```python
from build123d import *

# Parameters (mm, degrees)
SKETCH008_R          = 7.5
SKETCH008_R_2        = 6.6
PAD002_DEPTH         = 24
SKETCH009_R          = 9
SKETCH009_R_2        = 6.6
PAD003_DEPTH         = 2
POCKET006_DEPTH      = 81.774622
POCKET006_DEPTH_BACK = 81.774622
POLARPATTERN_COUNT   = 3


with BuildPart() as part:
    # Sketch008 (on DatumPlane) → Pad002 (new body)
    with BuildSketch(Plane.XZ.offset(50)):
        Circle(SKETCH008_R)
        Circle(SKETCH008_R_2, mode=Mode.SUBTRACT)
    extrude(amount=PAD002_DEPTH)

    # Sketch009 (on Face3 of Pad002) → Pad003 (join)
    with BuildSketch(Plane(origin=(0, -50, 0), x_dir=(1, 0, 0), z_dir=(0, 1, 0))):
        Circle(SKETCH009_R)
        Circle(SKETCH009_R_2, mode=Mode.SUBTRACT)
    extrude(amount=PAD003_DEPTH)

    # Sketch010 → Revolution (revolve)
    with BuildSketch(Plane.XY):
        Polygon((-7.5, -74), (-7.5, -71.3), (-8.7, -71.3), (-8.7, -72.3), (-7.7, -74), align=None)
    revolve(axis=Axis((0, 0, 0), (0, 1, 0)))

    # Sketch011 → Pocket006 (cut, two sides)
    with BuildSketch(Plane.XY) as pocket006_sk:
        with BuildLine():
            Line((-0.8, -74), (-0.8, -60))
            ThreePointArc((0.8, -60), (0, -59.2), (-0.8, -60))
            Line((0.8, -60), (0.8, -74))
            Line((-0.8, -74), (0.8, -74))
        make_face()
    pocket006 = extrude(amount=-POCKET006_DEPTH, mode=Mode.SUBTRACT) + extrude(pocket006_sk.sketch, amount=POCKET006_DEPTH_BACK, mode=Mode.SUBTRACT)

    # PolarPattern: Pocket006 ×3 about axis
    polarpattern_axis = Axis((0, 0, 0), (0, 1, 0))
    for i in range(1, POLARPATTERN_COUNT):
        add(pocket006.rotate(polarpattern_axis, i * 360 / POLARPATTERN_COUNT), mode=Mode.SUBTRACT)


solid = part.part
```
Geometry check sheet. Reference: the model listing, model coordinates, mm. A direction names the side the tool comes from. Round coordinates to 2 decimals unless told otherwise and drop trailing zeros. Order: outer loops, then holes, each group sorted by start corner. A loop starts at its lowest first (then second) coordinate and runs counter-clockwise, first axis right, second up. Notation, with made-up numbers: M 57.25,60 L 97.25,60 A26 ccw 97.25,86 Z; hole C 70,60 d7. An arc over 180 degrees is marked long. Write item = value, one per line.
Q1. Section check C-C (y = -64.25). Enter the section's corners in (x, z).
Answer block:
outline = M -6.86,-3.04 L -6.07,-2.58 A6.6 cw -6.07,2.58 L -6.86,3.04 A7.5 ccw Z; M -6.06,-4.42 A7.5 ccw -0.8,-7.46 L -0.8,-6.55 A6.6 cw -5.27,-3.97 Z; M -6.06,4.42 L -5.27,3.97 A6.6 cw -0.8,6.55 L -0.8,7.46 A7.5 ccw Z; M 0.8,-7.46 A7.5 ccw 6.06,-4.42 L 5.27,-3.97 A6.6 cw 0.8,-6.55 Z; M 0.8,6.55 A6.6 cw 5.27,3.97 L 6.06,4.42 A7.5 ccw 0.8,7.46 Z; M 6.07,-2.58 L 6.86,-3.04 A7.5 ccw 6.86,3.04 L 6.07,2.58 A6.6 cw Z
Q2. Set-up check for faces 5 (the flat face through (4, -71.3, -7)), 6 (the flat face through (-6.59, -68.46, -2.88)), 7 (the flat face through (0.8, -68, -7)): record each of +Z, -Z, +X, -X, +Y, -Y from which the full face is reachable in a straight line by a thin tool's end or side.
Answer block:
face_5 = -Z, +X
face_6 = -Y
face_7 = +Z, -Z, -Y
Q3. Section check D-D (y = -57). Enter the section's corners in (x, z), plus the area to 3 significant figures.
Answer block:
outline = C 0,0 d15; hole C 0,0 d13.2
area = 39.9 mm^2
Q4. Section check A-A (x = 0). Enter the section's corners in (y, z).
Answer block:
outline = M -59.2,-7.5 L -50,-7.5 L -50,-9 L -48,-9 L -48,-6.6 L -59.2,-6.6 Z; M -59.2,6.6 L -48,6.6 L -48,9 L -50,9 L -50,7.5 L -59.2,7.5 Z
Q5. Depth check by flat-ended pin: pin 1 Ø1.1 at (y, z) = (-67.5, -7.5) entering from +X; pin 2 Ø3 at (x, z) = (-2, -2.5) entering from -Y; pin 3 Ø1.7 at (y, z) = (-67.5, -7.5) entering from -X; pin 4 Ø8 at (x, y) = (6.5, -61.5) entering from -Z. Enter the tip coordinate at first touch or a pass-through.
Answer block:
pin_1 = 2.82
pin_2 = through
pin_3 = -3.47
pin_4 = -7.07
Q6. Release check for a two-part mould opening along Z. For faces 1 (the flat face through (-5.769, -68.654, 4.254)), 2 (the cylindrical face through (4.395, -71.807, -7.508)), 3 (the cylindrical face through (-4.395, -71.807, 7.508)), 4 (the flat face through (-0.8, -69, -7)) record: released by +Z, released by -Z, zero draft, split by the parting line, or undercut.
Answer block:
face_1 = undercut
face_2 = released by -Z
face_3 = released by +Z
face_4 = zero draft
Q7. Section check B-B (z = 0). Enter the section's corners in (x, y), plus the area to 3 significant figures.
Answer block:
outline = M -9,-50 L -7.5,-50 L -7.5,-71.3 L -8.7,-71.3 L -8.7,-72.3 L -7.7,-74 L -6.6,-74 L -6.6,-48 L -9,-48 Z; M 6.6,-74 L 7.7,-74 L 8.7,-72.3 L 8.7,-71.3 L 7.5,-71.3 L 7.5,-50 L 9,-50 L 9,-48 L 6.6,-48 Z
area = 57.6 mm^2
Q8. Scan lines: line 1 (X direction, y = -55, z = 0); line 2 (Z direction, x = 5.75, y = -54.25). Record each from-to range of solid material in increasing order.
Answer block:
line_1 = -7.5 to -6.6, 6.6 to 7.5
line_2 = -4.82 to -3.24, 3.24 to 4.82
